Input: part model. Units: mm. Frame: model coordinates. A direction names the side the tool comes from. Round coordinates to 2 decimals unless told otherwise and drop trailing zeros. Order: outer loops, then holes, each group sorted by start corner. A loop starts at its lowest first (then second) coordinate and runs counter-clockwise, first axis right, second up.
Item 1: First-contact query: pin 1 (8 mm diameter, centred on x = 18.5, y = 63, fed in from -Z). Flat tip, straight axial feed; report the tip coordinate or a pass-through.
Item 2: Cut plane C-C on x = 30. Output: boundary loops of the cut face in (y, z), then the cut area to 3 significant figures.
Item 3: Mould query, pull axis X, two halves, no side actions, for faces 3 (the flat face through (0, 25, -25.735)), 4 (the flat face through (3, 25, -64.382)), 5 (the flat face through (77.315, 25, -51)). Classes: released by +X, released by -X, zero draft, split by the parting line, or undercut.
Item 4: Cut plane A-A on z = -68.5. Output: boundary loops of the cut face in (x, y).
Item 5: Cut plane B-B on y = 33.5. Output: boundary loops of the cut face in (x, z).
Item 6: Line query: L1, parallel to Z at x = 16, y = -2; L2, parallel to Z at x = 49, y = 25; L3, parallel to Z at x = 46, y = 33. Output: solid intervals per line, ascending.
Item 7: Reachability of faces 1 (the flat face through (-36.95, 24.69, -76.25)), 2 (the flat face through (-55, 25, -76.535)) from +Z, -Z, +X, -X, +Y, -Y: full face, straight path, thin tool, end or side. Return the list, or none.
```python
from build123d import *

# Parameters (mm, degrees)
F0_W     = 152.4
F0_H     = 50.8
F1_DEPTH = 25.4
F4_DEPTH = 25.4
F5_DEPTH = 76.2


with BuildPart() as f1:
    # F0 (on Front) → F1 (new body)
    with BuildSketch(Plane.XZ):
        with Locations((1.1145584285, -51.1352052836)):
            Rectangle(F0_W, F0_H)
    extrude(amount=F1_DEPTH)

    # F3 (on face) → F4 (cut)
    with BuildSketch(Plane.XZ.offset(25.4)):
        Polygon((52.7703917205, -64.3824934959), (-48.8296082795, -64.3824934959), (-38.9320172776, -75.971078067), (-3.4057565499, -80.9468403459), (37.3732924352, -80.0572519513), (41.6376553476, -75.7159888744), align=None)
    extrude(amount=-F4_DEPTH, mode=Mode.SUBTRACT)

    # F5 (add): a face of the model
    f5_faces = [f1.faces().sort_by_distance(p)[0] for p in [
        (1.0289602376, 0, -47.9835586604),
    ]]
    extrude(f5_faces, amount=F5_DEPTH)


solid = f1.part
```
From the geometry:
1. pin 1: stops at z = -64.38
2. outline: (-25.4, -64.38) - (76.2, -64.38) - (76.2, -25.74) - (-25.4, -25.74) - close
2. area: 3,930 mm2
3. face 3: zero draft
3. face 4: undercut
3. face 5: released by +X
4. outline: (-75.09, -25.4) - (-45.31, -25.4) - (-45.31, 76.2) - (-75.09, 76.2) - close; (48.73, -25.4) - (77.31, -25.4) - (77.31, 76.2) - (48.73, 76.2) - close
5. outline: (-75.09, -76.54) - (-34.9, -76.54) - (-38.93, -75.97) - (-48.83, -64.38) - (52.77, -64.38) - (40.83, -76.54) - (77.31, -76.54) - (77.31, -25.74) - (-75.09, -25.74) - close
6. L1: z = -64.38 to -25.74
6. L2: z = -76.54 to -68.22, -64.38 to -25.74
6. L3: z = -76.54 to -71.27, -64.38 to -25.74
7. face 1: +Y, -Y
7. face 2: -Z, +X, -X, +Y, -Y
